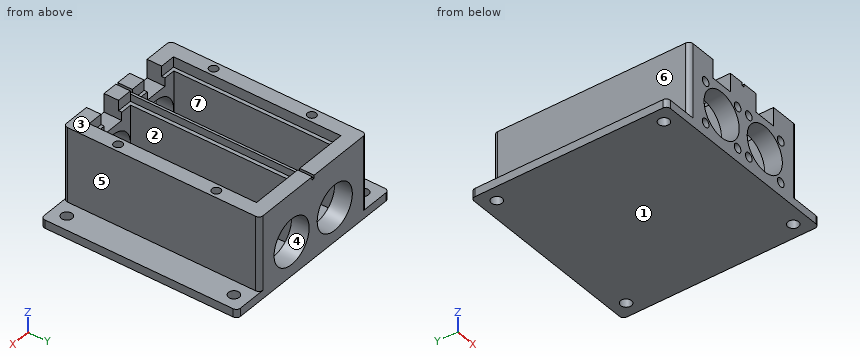
from build123d import *

# Parameters (mm, degrees)
PAD_DEPTH                     = 40
PAD001_DEPTH                  = 4
SKETCH002_W                   = 1.2
SKETCH002_H                   = 94.8
POCKET001_DEPTH               = 1.5
SKETCH003_W                   = 25.8
SKETCH003_H                   = 80.8
POCKET_DEPTH                  = 5
SKETCH004_W                   = 22.2
SKETCH004_H                   = 77.7
POCKET002_DEPTH               = 31
SKETCH005_R                   = 2.0955
POCKET003_DEPTH               = 7
SKETCH006_R                   = 11
POCKET004_DEPTH               = 374.955376
SKETCH010_W                   = 11
SKETCH010_H                   = 8.55
POCKET007_DEPTH               = 9
SKETCH009_R                   = 2.6035
POCKET006_DEPTH               = 40.001
SKETCH008_R                   = 2.0955
POCKET005_DEPTH               = 7
SKETCH008_MIRRORED004_2_R     = 2.0955
POCKET005_MIRRORED004_2_DEPTH = 7


with BuildPart() as part:
    # Sketch → Pad (new body)
    with BuildSketch(Plane.XY):
        with BuildLine():
            Line((-33.4, 45.4), (-33.4, -45.4))
            ThreePointArc((-33.4, -45.4), (-32.814214, -46.814214), (-31.4, -47.4))
            Line((-31.4, -47.4), (31.4, -47.4))
            ThreePointArc((31.4, -47.4), (32.814214, -46.814214), (33.4, -45.4))
            Line((33.4, -45.4), (33.4, 45.4))
            ThreePointArc((33.4, 45.4), (32.814214, 46.814214), (31.4, 47.4))
            Line((31.4, 47.4), (-31.4, 47.4))
            ThreePointArc((-31.4, 47.4), (-32.814214, 46.814214), (-33.4, 45.4))
        make_face()
    extrude(amount=PAD_DEPTH)

    # Sketch007 → Pad001 (join)
    with BuildSketch(Plane.XY):
        with BuildLine():
            Line((-47.5252, 45.4), (-47.5252, -45.4))
            ThreePointArc((-47.5252, -45.4), (-46.939414, -46.814214), (-45.5252, -47.4))
            Line((-45.5252, -47.4), (45.5252, -47.4))
            ThreePointArc((45.5252, -47.4), (46.939414, -46.814214), (47.5252, -45.4))
            Line((47.5252, -45.4), (47.5252, 45.4))
            ThreePointArc((47.5252, 45.4), (46.939414, 46.814214), (45.5252, 47.4))
            Line((45.5252, 47.4), (-45.5252, 47.4))
            ThreePointArc((-45.5252, 47.4), (-46.939414, 46.814214), (-47.5252, 45.4))
        make_face()
    extrude(amount=PAD001_DEPTH)

    # Sketch002 (on DatumPlane) → Pocket001 (cut)
    with BuildSketch(Plane.XY.offset(40)):
        Rectangle(SKETCH002_W, SKETCH002_H)
    extrude(amount=-POCKET001_DEPTH, mode=Mode.SUBTRACT)

    # Sketch003 (on DatumPlane) → Pocket (cut)
    with BuildSketch(Plane.XY.offset(40)):
        with Locations((-13.5, 0)):
            Rectangle(SKETCH003_W, SKETCH003_H)
    pocket = extrude(amount=-POCKET_DEPTH, mode=Mode.SUBTRACT)

    # Mirrored: Pocket across Sketch003 V_Axis
    add(pocket.mirror(Plane(origin=(0, 0, 40), x_dir=(0, 0, 1), z_dir=(1, 0, 0))), mode=Mode.SUBTRACT)

    # Sketch004 (on DatumPlane) → Pocket002 (cut)
    with BuildSketch(Plane.XY.offset(35)):
        with Locations((-13.5, 0)):
            Rectangle(SKETCH004_W, SKETCH004_H)
    pocket002 = extrude(amount=-POCKET002_DEPTH, mode=Mode.SUBTRACT)

    # Mirrored001: Pocket002 across Sketch004 V_Axis
    add(pocket002.mirror(Plane(origin=(0, 0, 35), x_dir=(0, 0, 1), z_dir=(1, 0, 0))), mode=Mode.SUBTRACT)

    # Sketch005 (on DatumPlane) → Pocket003 (cut)
    with BuildSketch(Plane.XZ.offset(47.4)):
        with Locations((-23.5, 26.5)):
            Circle(SKETCH005_R)
        with Locations((-3.5, 26.5)):
            Circle(SKETCH005_R)
        with Locations((-23.5, 6.5)):
            Circle(SKETCH005_R)
        with Locations((-3.5, 6.5)):
            Circle(SKETCH005_R)
    pocket003 = extrude(amount=-POCKET003_DEPTH, mode=Mode.SUBTRACT)

    # Mirrored002: Pocket003 across Sketch005 V_Axis
    add(pocket003.mirror(Plane(origin=(0, -47.4, 0), x_dir=(0, -1, 0), z_dir=(1, 0, 0))), mode=Mode.SUBTRACT)

    # Sketch006 (on DatumPlane) → Pocket004 (cut, through all)
    with BuildSketch(Plane.XZ.offset(47.4)):
        with Locations((-13.5, 16.5)):
            Circle(SKETCH006_R)
    pocket004 = extrude(amount=-POCKET004_DEPTH, mode=Mode.SUBTRACT)

    # Mirrored003: Pocket004 across Sketch006 V_Axis
    add(pocket004.mirror(Plane(origin=(0, -47.4, 0), x_dir=(0, -1, 0), z_dir=(1, 0, 0))), mode=Mode.SUBTRACT)

    # Sketch010 (on DatumPlane) → Pocket007 (cut)
    with BuildSketch(Plane.XY.offset(40)):
        with Locations((-13.5, -43.125)):
            Rectangle(SKETCH010_W, SKETCH010_H)
    pocket007 = extrude(amount=-POCKET007_DEPTH, mode=Mode.SUBTRACT)

    # Mirrored006: Pocket007 across Sketch010 V_Axis
    add(pocket007.mirror(Plane(origin=(0, 0, 40), x_dir=(0, 0, 1), z_dir=(1, 0, 0))), mode=Mode.SUBTRACT)

    # Sketch009 → Pocket006 (cut, through all)
    with BuildSketch(Plane.XY):
        with Locations((-40.4626, 40.3374)):
            Circle(SKETCH009_R)
        with Locations((40.4626, 40.3374)):
            Circle(SKETCH009_R)
        with Locations((-40.4626, -40.3374)):
            Circle(SKETCH009_R)
        with Locations((40.4626, -40.3374)):
            Circle(SKETCH009_R)
    extrude(amount=POCKET006_DEPTH, mode=Mode.SUBTRACT)

    # Sketch008 (on DatumPlane) → Pocket005 (cut)
    with BuildSketch(Plane.XY.offset(40)):
        with Locations((-29.9, 23.7)):
            Circle(SKETCH008_R)
    pocket005 = extrude(amount=-POCKET005_DEPTH, mode=Mode.SUBTRACT)

    # Sketch008 Mirrored004 2 → Pocket005 Mirrored004 2 (cut)
    with BuildSketch(Plane(origin=(0, 0, 40), x_dir=(-1, 0, 0), z_dir=(0, 0, -1))):
        with Locations((-29.9, 23.7)):
            Circle(SKETCH008_MIRRORED004_2_R)
    pocket005_mirrored004_2 = extrude(amount=POCKET005_MIRRORED004_2_DEPTH, mode=Mode.SUBTRACT)

    # Mirrored005: Pocket005, Pocket005 Mirrored004 2 across XZ
    add(pocket005.mirror(Plane.XZ), mode=Mode.SUBTRACT)
    add(pocket005_mirrored004_2.mirror(Plane.XZ), mode=Mode.SUBTRACT)


solid = part.part
The model under review builds one solid part; all positions refer to its coordinate system, in mm. Face numbers are marked on the shaded views. A direction names the side the tool comes from. Coordinates: 2 decimals unless noted, no trailing zeros. Loops run counter-clockwise (first coordinate to the right, second up) from the corner with the lowest first, then second, coordinate; pieces in that order, holes last. Notation, with made-up numbers: M 5,-40 L 55,-40 A13 cw 55,-19 Z; hole C 4,-26 d8. An arc over 180 degrees is marked long. Put each result on its own line as item: value. Start each with the question number.
Q1. Add section B-B (z = 20). Count the separate pieces of the cut face and the enclosed holes in it, and give its area (3 significant figures).
Q2. Add section A-A (x = -13.5). Write out the cut boundary in (y, z).
Q3. Add section C-C (y = 33). Write out the cut boundary in (x, z).
Q4. For the marked faces 5, 6 and 7, list the 3-axis set-ups (+Z, -Z, +X, -X, +Y, -Y) from which the entire face can be reached by the end or side of a thin tool; tool diameter is ignored.
Q5. Clearance check with flat-ended pins moving along their axes: pin 1 (4 mm diameter, centred on x = -29.9, y = 23.7, fed in from +Z); pin 2 (4 mm diameter, centred on y = -19, z = 38.5, fed in from -X); pin 3 (6.5 mm diameter, centred on x = 8.5, y = 5, fed in from +Z). State where each tip first meets the part, or that it passes through.
Q6. Wall thickness on line 1 (X direction, y = -4, z = 29); line 2 (X direction, y = 42, z = 16); line 3 (Z direction, x = -13, y = 44): over which ranges is each line inside the solid? List them lowest first.
Q7. The part is to be moulded in two halves that separate along Z. For the marked faces 1, 2, 3 and 4, say which applies: +Z half, -Z half, draft (parallel to the pull), parting line (faces both ways), or undercut.
Answers:
1. separate pieces: 3
1. enclosed holes: 0
1. area: 2,170 mm^2
2. outline: M -47.4,0 L 47.4,0 L 47.4,5.5 L 38.85,5.5 L 38.85,4 L -38.85,4 L -38.85,5.5 L -47.4,5.5 Z; M -47.4,27.5 L -38.85,27.5 L -38.85,31 L -47.4,31 Z; M 38.85,27.5 L 47.4,27.5 L 47.4,40 L 40.4,40 L 40.4,35 L 38.85,35 Z
3. outline: M -47.53,0 L 47.53,0 L 47.53,4 L 33.4,4 L 33.4,40 L 26.4,40 L 26.4,35 L 24.6,35 L 24.6,4 L 2.4,4 L 2.4,35 L 0.6,35 L 0.6,38.5 L -0.6,38.5 L -0.6,35 L -2.4,35 L -2.4,4 L -24.6,4 L -24.6,35 L -26.4,35 L -26.4,40 L -33.4,40 L -33.4,4 L -47.53,4 Z
4. face 5: +Z, +X, +Y, -Y
4. face 6: +Z, -X, +Y, -Y
4. face 7: +Z
5. pin 1: stops at z = 33
5. pin 2: stops at x = -33.4
5. pin 3: stops at z = 4
6. line 1: x = -33.4 to -24.6, -2.4 to 2.4, 24.6 to 33.4
6. line 2: x = -33.4 to -24.49, -2.51 to 2.51, 24.49 to 33.4
6. line 3: z = 0 to 5.51, 27.49 to 40
7. face 1: -Z half
7. face 2: draft
7. face 3: +Z half
7. face 4: undercut
